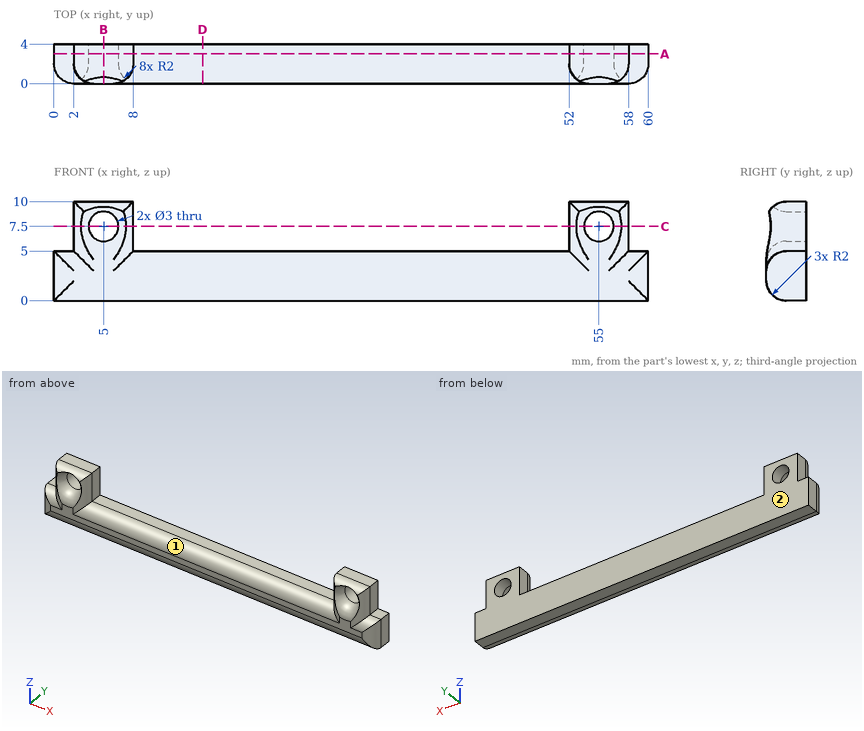
Could you check a few things on this drawing? It's one solid part, dimensions in mm from its lowest x, y, z. A direction names the side the tool comes from. Coordinates: 2 decimals unless noted, no trailing zeros. Loops run counter-clockwise (first coordinate to the right, second up) from the corner with the lowest first, then second, coordinate; pieces in that order, holes last. Notation, with made-up numbers: (6.25, -31) - (22.25, -31) arc R21 ccw to (22.25, 4) - close; hole circle Ø10 at (9, 84.5). An arc over 180 degrees is marked (long way). Return JSON: item names as keys, results as strings. Group by question number.
Item 1: If we section it at B-B on x = 5: Write out the boundary of the cut face in (y, z), and give its area (3 significant figures).
Item 2: If we section it at D-D on x = 15: Write out the boundary of the cut face in (y, z), and give its area (3 significant figures).
Item 3: Will these pins go through, and if not, where does the flat tip stop? P1, Ø0.6, axis at y = 2.5, z = 6.5, coming from the +X side; P2, Ø1.5, axis at y = 0.5, z = 9, coming from the +X side; P3, Ø4, axis at x = 55, z = 7.5, coming from the -Y side.
Item 4: If we section it at C-C on z = 7.5: Write out the boundary of the cut face in (x, y), and give its area (3 significant figures).
Item 5: If we section it at A-A on y = 3: Write out the boundary of the cut face in (x, z).
Item 6: On a 3-axis mill with a long thin cutter (end or side, diameter ignored), from which of +Z, -Z, +X, -X, +Y, -Y can I reach the whole of each face in a straight line? I mean the marked faces 1 and 2. Say none if no direction works.
Item 7: I need wall thicknesses on line 1 (Z direction, x = 5, y = 2.6); line 2 (X direction, y = 2.35, z = 8); line 3 (X direction, y = 2.85, z = 6.5). Which ranges of each line are inside material? Lowest first, please. Write a range as from..to.
Calculated:
{
 "1": {"outline": "(0, 2) arc R2 ccw to (2, 0) - (4, 0) - (4, 6) - (2, 6) arc R2 ccw to (0, 4) - close; (0.68, 9.5) arc R2 ccw to (2, 9) - (4, 9) - (4, 10) - (2, 10) arc R2 ccw to start", "area": "25.2 mm^2"},
 "2": {"outline": "(0, 2) arc R2 ccw to (2, 0) - (4, 0) - (4, 5) - (2, 5) arc R2 ccw to (0, 3) - close", "area": "18.3 mm^2"},
 "3": {"P1": "stops at x = 58", "P2": "stops at x = 57.85", "P3": "stops at y = 0.68"},
 "4": {"outline": "(2, 2) arc R2 ccw to (2.75, 0.44) arc R2 ccw to (3.5, 2) - (3.5, 4) - (2, 4) - close; (6.5, 2) arc R2 ccw to (7.25, 0.44) arc R2 ccw to (8, 2) - (8, 4) - (6.5, 4) - close; (52, 2) arc R2 ccw to (52.75, 0.44) arc R2 ccw to (53.5, 2) - (53.5, 4) - (52, 4) - close; (56.5, 2) arc R2 ccw to (57.25, 0.44) arc R2 ccw to (58, 2) - (58, 4) - (56.5, 4) - close", "area": "18.5 mm^2"},
 "5": {"outline": "(0, 0) - (60, 0) - (60, 5) - (58, 5) - (58, 10) - (52, 10) - (52, 5) - (8, 5) - (8, 10) - (2, 10) - (2, 5) - (0, 5) - close; hole circle Ø3 at (5, 7.5); hole circle Ø3 at (55, 7.5)"},
 "6": {"face 1": "+Z, -Y", "face 2": "+Z, -Z, +X, -X, +Y"},
 "7": {"line 1": "z = 0..6, 9..10", "line 2": "x = 2..3.59, 6.41..8, 52..53.59, 56.41..58", "line 3": "x = 2..3.88, 6.12..8, 52..53.88, 56.12..58"}
}
